Geometry check sheet. Reference: the model listing, model coordinates, mm. A direction names the side the tool comes from. Give positions to 0.01 mm unless a question says otherwise; leave off trailing zeros. Loops run counter-clockwise (first coordinate to the right, second up) from the corner with the lowest first, then second, coordinate; pieces in that order, holes last.
1. Cross-section at A-A, the plane x = -9.5. Record the cut outline in (y, z).
2. Cross-section at D-D, the plane x = 4. Record the cut outline in (y, z).
3. Release check for a two-part mould opening along X. For faces 1 (the flat face through (-12, 8.3, 25.2)), 2 (the flat face through (-6, 0, 87)), 3 (the flat face through (6, 0, 87)), 4 (the flat face through (9.465, 13.184, 30.21)) record: +X half, -X half, draft (parallel to the pull), parting line (faces both ways), or undercut.
4. Material ranges on L1, parallel to X at y = -1, z = 56.5; L2, parallel to Y at x = 10.25, z = 11; L3, parallel to X at y = -9, z = 26, recorded low to high.
5. Tool access check on faces 5 (the flat face through (-9, -14, 0)), 6 (the flat face through (9, 10, -2)), 7 (the cylindrical face through (9.46, 9.31, 11.43)), 8 (the cylindrical face through (-9.5, 3.9, 2.6)), 9 (the flat face through (-7, 0, 145)). Record the directions out of +Z, -Z, +X, -X, +Y, -Y that give a thin tool (end or side, any length) a straight path to the whole face; none if there is none.
6. Go/stop test with flat-tipped pins: pin 1 Ø4.5 at (x, z) = (-3, 84) entering from +Y; pin 2 Ø1.5 at (x, y) = (-8.5, 13) entering from -Z; pin 3 Ø4.5 at (x, z) = (0, 97.5) entering from -Y; pin 4 Ø12 at (y, z) = (0, 15) entering from +X. Record where each tip stops, or that it passes through.
7. Cross-section at B-B, the plane z = 135. Record the cut outline in (x, y), plus the area to 3 significant figures.
8. Cross-section at C-C, the plane y = -14.5. Record the cut outline in (x, z).
from build123d import *

# Parameters (mm, degrees)
SKETCH_3_R           = 6.6
SKETCH_3_R_2         = 1.6
EXTRUDE_1_DEPTH      = 5
SKETCH_5_R           = 13
EXTRUDE_2_DEPTH      = 5
EXTRUDE_3_DEPTH      = 100
EXTRUDE_3_DEPTH_BACK = 15
SKETCH_6_W           = 15
SKETCH_6_H           = 15
SKETCH_6_W_2         = 12
SKETCH_6_H_2         = 12
SKETCH_7_R           = 4
CUT_EXTRUDE_1_DEPTH  = 148.408446162


with BuildPart() as part:
    # Sketch 3 → Extrude 1 (new body)
    with BuildSketch(Plane(origin=(7, 0, 0), x_dir=(0, 0, -1), z_dir=(1, 0, 0))):
        Polygon((5, 10), (5, -10), (0, -10), (0, -18), (-15, -18), (-45, -8.5), (-45, 8.5), (-15, 18), (0, 18), (0, 10), align=None)
        with Locations((-15, 0)):
            Circle(SKETCH_3_R, mode=Mode.SUBTRACT)
        with Locations((-24.5, 0)):
            Circle(SKETCH_3_R_2, mode=Mode.SUBTRACT)
        with Locations((-10.25, 8.227241336)):
            Circle(SKETCH_3_R_2, mode=Mode.SUBTRACT)
        with Locations((-10.25, -8.227241336)):
            Circle(SKETCH_3_R_2, mode=Mode.SUBTRACT)
    extrude(amount=EXTRUDE_1_DEPTH)



with BuildPart() as body_2:
    # Sketch 5 → Extrude 2 (new body)
    with BuildSketch(Plane(origin=(-7, 0, 0), x_dir=(0, 0, -1), z_dir=(1, 0, 0))):
        Polygon((-45, -8.5), (-45, 8.5), (-15, 18), (0, 18), (0, 10), (5, 10), (5, -10), (0, -10), (0, -18), (-15, -18), align=None)
        with Locations((-15, 0)):
            Circle(SKETCH_5_R, mode=Mode.SUBTRACT)
    extrude(amount=-EXTRUDE_2_DEPTH)


with BuildPart() as part_1:
    add(part.part)

    add(body_2.part)  # Extrude 3 merges body 2
    # Sketch 6 → Extrude 3 (add, two sides: drawn at the far end of the back side and taken through both)
    with BuildSketch(Plane.XY.offset(45).offset(-EXTRUDE_3_DEPTH_BACK)):
        Rectangle(SKETCH_6_W, SKETCH_6_H)
        Rectangle(SKETCH_6_W_2, SKETCH_6_H_2, mode=Mode.SUBTRACT)
    extrude(amount=EXTRUDE_3_DEPTH + EXTRUDE_3_DEPTH_BACK)

    # Sketch 7 → Cut-Extrude 1 (cut, through all)
    with BuildSketch(Plane(origin=(7.5, 0, 0), x_dir=(0, 0, -1), z_dir=(1, 0, 0))):
        with Locations((-135, 0)):
            Circle(SKETCH_7_R)
    extrude(amount=-CUT_EXTRUDE_1_DEPTH, mode=Mode.SUBTRACT)


solid = part_1.part
Result:
1. outline: (-18, 0) - (-10, 0) - (-10, -5) - (10, -5) - (10, 0) - (18, 0) - (18, 15) - (8.5, 45) - (-8.5, 45) - (-18, 15) - close; hole circle Ø26 at (0, 15)
2. outline: (-7.5, 30) - (-6, 30) - (-6, 145) - (-7.5, 145) - close; (6, 30) - (7.5, 30) - (7.5, 145) - (6, 145) - close
3. face 1: -X half
3. face 2: undercut
3. face 3: undercut
3. face 4: draft
4. L1: x = -7.5 to -6, 6 to 7.5
4. L2: y = -18 to -9.64, -6.81 to -5.25, 5.25 to 6.81, 9.64 to 18
4. L3: x = -12 to -7, 7 to 12
5. face 5: -Z, +X, -X, -Y
5. face 6: -Z, +X, -X, +Y
5. face 7: +X, -X
5. face 8: -X
5. face 9: +Z, +X, -X, +Y, -Y
6. pin 1: stops at y = 7.5
6. pin 2: stops at z = 0
6. pin 3: stops at y = -7.5
6. pin 4: passes through
7. outline: (-7.5, -7.5) - (7.5, -7.5) - (7.5, -4) - (6, -4) - (6, -6) - (-6, -6) - (-6, -4) - (-7.5, -4) - close; (-7.5, 4) - (-6, 4) - (-6, 6) - (6, 6) - (6, 4) - (7.5, 4) - (7.5, 7.5) - (-7.5, 7.5) - close
7. area: 57.0 mm2
8. outline: (-12, 0) - (-7, 0) - (-7, 26.05) - (-12, 26.05) - close; (7, 0) - (12, 0) - (12, 26.05) - (7, 26.05) - close
